Input: part model. Units: mm. Frame: model coordinates. Face numbers are marked on the shaded views. A direction names the side the tool comes from. Coordinates: 2 decimals unless noted, no trailing zeros. Write each loop counter-clockwise with the first axis right and the second up, starting at its lowest first coordinate (ties: lowest second). Pieces come first, ordered by that corner, then holes. Notation, with made-up numbers: (-24, 13) -> (-7, 13) arc R25 cw to (-7, 27) -> close; hole circle Ø6 at (51, 22). An arc over 180 degrees is marked (long way). Use one line per item in the form item = value. Start each with the question number.
(1) Ray query, line 1 along X through (y, z) = (1.15, 0.75); line 2 along X through (y, z) = (0.15, 1.55); line 3 along Z through (x, y) = (1, -1). Return the intervals inside material, ascending.
(2) Cut plane B-B on x = 3.5. Return the cut outline in (y, z).
(3) Pull-direction query (X, two-part tool) for the marked faces 4, 5 and 6; classes: released by +X, released by -X, zero draft, split by the parting line, or undercut.
(4) Cut plane A-A on x = 2.25. Return the cut outline in (y, z), plus the area to 3 significant figures.
(5) First-contact query: pin 1 (1.5 mm diameter, centred on x = 5.5, z = 1, fed in from +Y); pin 2 (2 mm diameter, centred on x = 2.5, z = 1, fed in from -Y); pin 3 (1 mm diameter, centred on y = -1.5, z = 1.5, fed in from +X). Flat tips, straight axial feed; report the tip coordinate or a pass-through.
(6) Set-up query: the marked faces 1, 2 and 3. Return all of +Z, -Z, +X, -X, +Y, -Y with unobstructed straight access to the full face (end or side cutting, diameter ignored); none if empty.
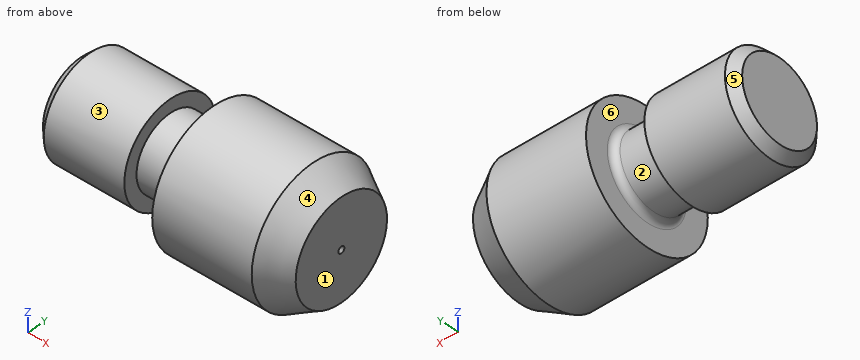
```python
from build123d import *

# Parameters (mm, degrees)
CHAMFER5_SIZE = 0.2705


with BuildPart() as part:
    # Sketch1 → Revolve1 (revolve)
    with BuildSketch(Plane.XY, mode=Mode.PRIVATE) as revolve1_sk:
        with BuildLine():
            Line((0, 0), (0, 1.5))
            Line((0, 1.5), (2.7, 1.5))
            Line((2.7, 1.5), (2.7, 1.1))
            Line((2.7, 1.1), (3.8, 1.1))
            ThreePointArc((3.8, 1.1), (3.941421356, 1.158578644), (4, 1.3))
            Line((4, 1.3), (4, 2))
            Line((4, 2), (7, 2))
            Line((7, 2), (7, 0))
            Line((7, 0), (0, 0))
        make_face()
    revolve(revolve1_sk.sketch.rotate(Axis((0, 0, 0), (1, 0, 0)), 90), axis=Axis((0, 0, 0), (1, 0, 0)))

    # Chamfer5
    chamfer5_edges = [part.edges().sort_by_distance(p)[0] for p in [
        (0, 0, -1.5),
    ]]
    chamfer(chamfer5_edges, length=CHAMFER5_SIZE)

    # Sketch5 → Revolve3 (revolve)
    with BuildSketch(Plane.XY, mode=Mode.PRIVATE) as revolve3_sk:
        Polygon((7, 0), (7, 2), (7.866025404, 1.5), (7.866025404, 0), align=None)
    revolve(revolve3_sk.sketch.rotate(Axis((0, 0, 0), (1, 0, 0)), 270), axis=Axis((0, 0, 0), (1, 0, 0)))

    # Sketch6 → Cut-Revolve3 (revolve, cut)
    with BuildSketch(Plane.XY, mode=Mode.PRIVATE) as cut_revolve3_sk:
        Polygon((7.866025404, 0.1), (7.866025404, 0), (7.766025404, 0), align=None)
    revolve(cut_revolve3_sk.sketch.rotate(Axis((0, 0, 0), (1, 0, 0)), 270), axis=Axis((0, 0, 0), (1, 0, 0)), mode=Mode.SUBTRACT)


solid = part.part
```
Values:
q1.line_1 = 0.14 to 2.7, 4 to 7.87
q1.line_2 = 4 to 7.77
q1.line_3 = -1.12 to 1.12
q2.outline = circle Ø2.2 at (0, 0)
q3.face_4 = released by +X
q3.face_5 = released by -X
q3.face_6 = undercut
q4.outline = circle Ø3 at (0, 0)
q4.area = 7.07 mm2
q5.pin_1 = 1.98
q5.pin_2 = -1.5
q5.pin_3 = 7.66
q6.face_1 = +Z, -Z, +X, +Y, -Y
q6.face_2 = none
q6.face_3 = -X
